```python
from build123d import *

# Parameters (mm, degrees)
SKIZZE1_W                                            = 80
SKIZZE1_H                                            = 120
AUFSATZ_LINEAR_AUSTRAGEN1_DEPTH                      = 6
FORMSENKUNG_F_R_M4_SENKSCHRAUBE_MIT_INNE_D           = 4.3
FORMSENKUNG_F_R_M4_SENKSCHRAUBE_MIT_INNE_DEPTH       = 11.5
FORMSENKUNG_F_R_M4_SENKSCHRAUBE_MIT_INNE_CSINK_D     = 9.18
FORMSENKUNG_F_R_M4_SENKSCHRAUBE_MIT_INNE_CSINK_ANGLE = 90
FORMSENKUNG_F_R_M4_SENKSCHRAUBE_MIT_INNE_TIP         = 1.291850331
F_3_0MM_STIFTLOCH1_D                                 = 3
F_3_0MM_STIFTLOCH1_DEPTH                             = 11.5
F_3_0MM_STIFTLOCH1_TIP                               = 0.901290929
STIRNSENKUNG_F_R_M3_FLACHKOPFSCHRAUBE_MI_D           = 3.4
STIRNSENKUNG_F_R_M3_FLACHKOPFSCHRAUBE_MI_DEPTH       = 8.5
STIRNSENKUNG_F_R_M3_FLACHKOPFSCHRAUBE_MI_CBORE_D     = 7
STIRNSENKUNG_F_R_M3_FLACHKOPFSCHRAUBE_MI_CBORE_DEPTH = 2.4
STIRNSENKUNG_F_R_M3_FLACHKOPFSCHRAUBE_MI_TIP         = 1.021463052
M10_GEWINDEBOHRUNG1_D                                = 8.5
SKIZZE28_W                                           = 40
SKIZZE28_H                                           = 35
SKIZZE28_H_2                                         = 15
SCHNITT_LINEAR_AUSTRAGEN1_DEPTH                      = 10
M4_GEWINDEBOHRUNG1_D                                 = 3.3
M4_GEWINDEBOHRUNG1_CSINK_D                           = 4.05
M4_GEWINDEBOHRUNG1_CSINK_ANGLE                       = 90
VERRUNDUNG1_R                                        = 5


with BuildPart() as part:
    # Skizze1 → Aufsatz-Linear austragen1 (new body)
    with BuildSketch(Plane.XY.offset(10)):
        with Locations((-40, 60)):
            Rectangle(SKIZZE1_W, SKIZZE1_H)
    extrude(amount=-AUFSATZ_LINEAR_AUSTRAGEN1_DEPTH)

    # Formsenkung für M4 Senkschraube mit Innensechskant1
    with Locations(Plane.XY.offset(10)):
        with Locations((-46, 60), (-15, 60)):
            CounterSinkHole(FORMSENKUNG_F_R_M4_SENKSCHRAUBE_MIT_INNE_D / 2, FORMSENKUNG_F_R_M4_SENKSCHRAUBE_MIT_INNE_CSINK_D / 2, depth=FORMSENKUNG_F_R_M4_SENKSCHRAUBE_MIT_INNE_DEPTH, counter_sink_angle=FORMSENKUNG_F_R_M4_SENKSCHRAUBE_MIT_INNE_CSINK_ANGLE)
            with Locations((0, 0, -(FORMSENKUNG_F_R_M4_SENKSCHRAUBE_MIT_INNE_DEPTH + FORMSENKUNG_F_R_M4_SENKSCHRAUBE_MIT_INNE_TIP / 2))):  # 118° drill point
                Cone(0, FORMSENKUNG_F_R_M4_SENKSCHRAUBE_MIT_INNE_D / 2, FORMSENKUNG_F_R_M4_SENKSCHRAUBE_MIT_INNE_TIP, mode=Mode.SUBTRACT)

    # Ø3.0mm Stiftloch1
    with Locations(Plane.XY.offset(10)):
        with Locations((-46, 74), (-15, 74), (-15, 46), (-46, 46)):
            Hole(F_3_0MM_STIFTLOCH1_D / 2, depth=F_3_0MM_STIFTLOCH1_DEPTH)
            with Locations((0, 0, -(F_3_0MM_STIFTLOCH1_DEPTH + F_3_0MM_STIFTLOCH1_TIP / 2))):  # 118° drill point
                Cone(0, F_3_0MM_STIFTLOCH1_D / 2, F_3_0MM_STIFTLOCH1_TIP, mode=Mode.SUBTRACT)

    # Stirnsenkung für M3 Flachkopfschraube mit Schlitz2
    with Locations(Plane(origin=(0, 0, 4), x_dir=(-1, 0, 0), z_dir=(0, 0, -1))):
        with Locations((25, 112.5), (25, 97.5), (5, 97.5), (5, 112.5), (25, 22.5), (25, 7.5), (5, 7.5), (5, 22.5)):
            CounterBoreHole(STIRNSENKUNG_F_R_M3_FLACHKOPFSCHRAUBE_MI_D / 2, STIRNSENKUNG_F_R_M3_FLACHKOPFSCHRAUBE_MI_CBORE_D / 2, STIRNSENKUNG_F_R_M3_FLACHKOPFSCHRAUBE_MI_CBORE_DEPTH, depth=STIRNSENKUNG_F_R_M3_FLACHKOPFSCHRAUBE_MI_DEPTH)
            with Locations((0, 0, -(STIRNSENKUNG_F_R_M3_FLACHKOPFSCHRAUBE_MI_DEPTH + STIRNSENKUNG_F_R_M3_FLACHKOPFSCHRAUBE_MI_TIP / 2))):  # 118° drill point
                Cone(0, STIRNSENKUNG_F_R_M3_FLACHKOPFSCHRAUBE_MI_D / 2, STIRNSENKUNG_F_R_M3_FLACHKOPFSCHRAUBE_MI_TIP, mode=Mode.SUBTRACT)

    # M10 Gewindebohrung1 (through all)
    with Locations(Plane(origin=(0, 0, 4), x_dir=(-1, 0, 0), z_dir=(0, 0, -1))):
        with Locations((45, 30)):
            Hole(M10_GEWINDEBOHRUNG1_D / 2)

    # Skizze28 → Schnitt-Linear austragen1 (cut)
    with BuildSketch(Plane(origin=(0, 0, 4), x_dir=(-1, 0, 0), z_dir=(0, 0, -1))):
        with Locations((60, 102.5)):
            Rectangle(SKIZZE28_W, SKIZZE28_H)
        with Locations((60, 7.5)):
            Rectangle(SKIZZE28_W, SKIZZE28_H_2)
    extrude(amount=-SCHNITT_LINEAR_AUSTRAGEN1_DEPTH, mode=Mode.SUBTRACT)

    # M4 Gewindebohrung1 (through all)
    with Locations(Plane(origin=(0, 0, 4), x_dir=(-1, 0, 0), z_dir=(0, 0, -1))):
        with Locations((65, 30)):
            CounterSinkHole(M4_GEWINDEBOHRUNG1_D / 2, M4_GEWINDEBOHRUNG1_CSINK_D / 2, counter_sink_angle=M4_GEWINDEBOHRUNG1_CSINK_ANGLE)

    # Verrundung1
    verrundung1_edges = [part.edges().sort_by_distance(p)[0] for p in [
        (-40, 85, 7),
        (-40, 15, 7),
    ]]
    fillet(verrundung1_edges, radius=VERRUNDUNG1_R)


solid = part.part
```
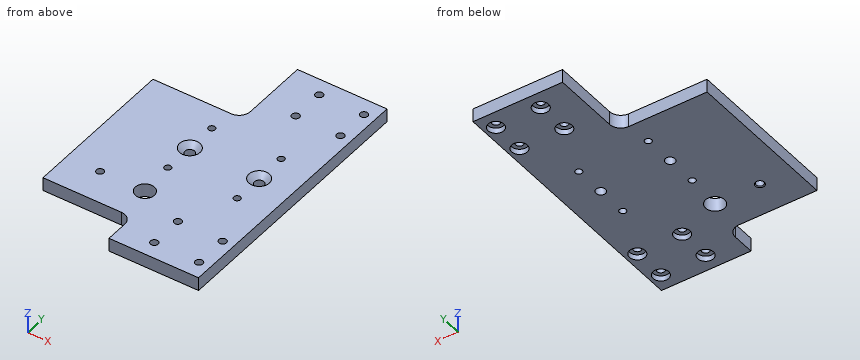
Design review of the part built by this model. Coordinates are the model's own, in mm. Give positions to 0.01 mm unless a question says otherwise; leave off trailing zeros. Order: outer loops, then holes, each group sorted by start corner. A loop starts at its lowest first (then second) coordinate and runs counter-clockwise, first axis right, second up. Notation, with made-up numbers: (1, 58.25) -> (58, 58.25) arc R29 cw to (58, 78.25) -> close; hole circle Ø1 at (12, 47.5). An arc over 180 degrees is marked (long way). Write each question's results on one line, items separated by ' | '. Start each with the question number.
Q1. Add section C-C on y = 112.5. Give the boundary of the cut face in (x, z).
Q2. For pin 1 (3 mm diameter, centred on x = -69, z = 8.5, fed in from -Y); pin 2 (2 mm diameter, centred on x = -69, z = 7, fed in from +Y); pin 3 (4.5 mm diameter, centred on x = -5, y = 97.5, fed in from -Z), all flat-tipped, find the tip position at first contact; note any pin that passes through.
Q3. Wall thickness on L1, parallel to Y at x = -25, z = 4.85; L2, parallel to Y at x = -65, z = 7.2; L3, parallel to Y at x = -15, z = 6.35: over which ranges is each line inside the solid? List them lowest first. Write a range as from..to.
Q4. Add section D-D on x = -5. State how many separate pieces and enclosed holes the cut face has, and give its area (3 significant figures).
Q5. Add section B-B on x = -15. Give the boundary of the cut face in (y, z), and give its area (3 significant figures).
Q6. Add section A-A on y = 30. Give the boundary of the cut face in (x, z) (3 decimals).
Found:
1) outline: (-40, 4) -> (-28.5, 4) -> (-28.5, 6.4) -> (-26.7, 6.4) -> (-26.7, 10) -> (-40, 10) -> close; (-23.3, 6.4) -> (-21.5, 6.4) -> (-21.5, 4) -> (-8.5, 4) -> (-8.5, 6.4) -> (-6.7, 6.4) -> (-6.7, 10) -> (-23.3, 10) -> close; (-3.3, 6.4) -> (-1.5, 6.4) -> (-1.5, 4) -> (0, 4) -> (0, 10) -> (-3.3, 10) -> close
2) pin 1: stops at y = 15 | pin 2: stops at y = 85 | pin 3: stops at z = 6.4
3) L1: y = 0..4, 11..19, 26..94, 101..109, 116..120 | L2: y = 15..28.35, 31.65..85 | L3: y = 0..44.5, 47.5..57.85, 62.15..72.5, 75.5..120
4) separate pieces: 5 | enclosed holes: 0 | area: 604 mm2
5) outline: (0, 4) -> (44.5, 4) -> (44.5, 10) -> (0, 10) -> close; (47.5, 4) -> (57.85, 4) -> (57.85, 7.56) -> (55.41, 10) -> (47.5, 10) -> close; (62.15, 4) -> (72.5, 4) -> (72.5, 10) -> (64.59, 10) -> (62.15, 7.56) -> close; (75.5, 4) -> (120, 4) -> (120, 10) -> (75.5, 10) -> close | area: 652 mm2
6) outline: (-80, 4) -> (-67.025, 4) -> (-66.65, 4.375) -> (-66.65, 10) -> (-80, 10) -> close; (-63.35, 4.375) -> (-62.975, 4) -> (-49.25, 4) -> (-49.25, 10) -> (-63.35, 10) -> close; (-40.75, 4) -> (0, 4) -> (0, 10) -> (-40.75, 10) -> close
